```python
from build123d import *

# Parameters (mm, degrees)
F0_W      = 2.2
F0_H      = 15
F1_DEPTH  = 1.5
F0_W_2    = 4.4
F0_H_2    = 4.6
F2_DEPTH  = 15
F3_SIZE   = 12
F5_DEPTH  = 25
F6_R      = 2.85
F7_DEPTH  = 2.2
F8_R      = 1.2
F9_R      = 7.49999
F10_R     = 3.35
F11_DEPTH = 25


# Not quite as in the source:
# - a fillet or chamfer is up to 0.001 mm smaller than in the source, because OpenCascade refuses the exact size
# - a pattern or mirror of a feature is missing from the dataset's text; its kind, count and spacing are read off the source's solid


with BuildPart() as f1:
    # F0 (on Top) → F1 (new body)
    with BuildSketch(Plane.XY):
        Polygon((8.1, 0.4), (8.1, 5), (-8.1, 5), (-8.1, 0.4), (-8.1, -5), (-8.1, -20), (8.1, -20), (8.1, -5), align=None)
        with Locations((-9.2, -12.5)):
            Rectangle(F0_W, F0_H)
        with Locations((9.2, -12.5)):
            Rectangle(F0_W, F0_H)
    extrude(amount=F1_DEPTH)

    # F0 (on Top) → F2 (join)
    with BuildSketch(Plane.XY):
        with Locations((-10.3, 12.5)):
            Rectangle(F0_W_2, F0_H)
        with Locations((10.3, 12.5)):
            Rectangle(F0_W_2, F0_H)
        with Locations((-10.3, 2.7)):
            Rectangle(F0_W_2, F0_H_2)
        with Locations((10.3, 2.7)):
            Rectangle(F0_W_2, F0_H_2)
        with Locations((-11.4, -12.5)):
            Rectangle(F0_W, F0_H)
        Polygon((-8.1, -5), (-8.1, 0.4), (-12.5, 0.4), (-12.5, -5), (-10.3, -5), align=None)
        Polygon((12.5, -5), (12.5, 0.4), (8.1, 0.4), (8.1, -5), (10.3, -5), align=None)
        with Locations((11.4, -12.5)):
            Rectangle(F0_W, F0_H)
    extrude(amount=F2_DEPTH)

    # F3
    f3_edges = [f1.edges().sort_by_distance(p)[0] for p in [
        (11.4, -20, 15),
        (-11.4, -20, 15),
    ]]
    chamfer(f3_edges, length=F3_SIZE)

    # F4 (on face) → F5 (cut)
    with BuildSketch(Plane.YZ.offset(12.5)):
        Polygon((6, 12.653529644), (5, 15), (0.3, 15), (-0.7, 12.653529644), align=None)
    extrude(amount=-F5_DEPTH, mode=Mode.SUBTRACT)

    # F6 (on face) → F7 (cut)
    with BuildSketch(Plane.YZ.offset(-8.1)):
        with BuildLine():
            Line((20, 1.3383538289), (20, 13.6716461711))
            ThreePointArc((20, 13.6716461711), (19.1242226672, 14.3975416295), (18.1593630584, 15))
            Line((18.1593630584, 15), (10.1406412151, 15))
            ThreePointArc((10.1406412151, 15), (5.6500087774, 7.4943749708), (10.1593912813, 0))
            Line((10.1593912813, 0), (18.1406129922, 0))
            ThreePointArc((18.1406129922, 0), (19.1156030804, 0.6062459626), (20, 1.3383538289))
        make_face()
        with Locations((14.1500021368, 7.505)):
            Circle(F6_R, mode=Mode.SUBTRACT)
    f7 = extrude(amount=-F7_DEPTH, mode=Mode.SUBTRACT)

    # F7_copies: F7 across plane
    add(f7.mirror(Plane(origin=(0, 0, 0), x_dir=(0, 0, 1), z_dir=(1, 0, 0))), mode=Mode.SUBTRACT)

    # F8
    f8_edges = [f1.edges().sort_by_distance(p)[0] for p in [
        (-8.1, 11.300002, 7.505),
        (8.1, 11.300002, 7.505),
    ]]
    fillet(f8_edges, radius=F8_R)

    # F9 (radius 7.5 in the source; OpenCascade refuses exactly that, so slightly less here)
    f9_edges = [f1.edges().sort_by_distance(p)[0] for p in [
        (-10.3, 20, 15),
        (-10.3, 20, 0),
        (10.3, 20, 15),
        (10.3, 20, 0),
    ]]
    fillet(f9_edges, radius=F9_R)

    # F10 (on face) → F11 (cut)
    with BuildSketch(Plane.XY.offset(1.5)):
        with Locations((0, -12)):
            Circle(F10_R)
    extrude(amount=-F11_DEPTH, mode=Mode.SUBTRACT)


solid = f1.part
```
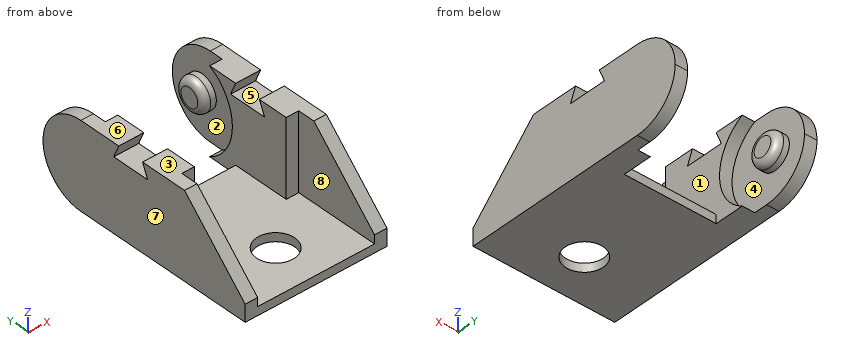
Check sheet for the modelled part. Datum: model origin and axes. Units: mm. Face numbers are marked on the shaded views. A direction names the side the tool comes from. Coordinates: 2 decimals unless noted, no trailing zeros. Loops run counter-clockwise (first coordinate to the right, second up) from the corner with the lowest first, then second, coordinate; pieces in that order, holes last.
1) Sectioned sample at B-B (y = -2.5). Record the boundary of the cut face in (x, z), and give its area (3 significant figures).
2) Sectioned sample at A-A (x = 0). Record the boundary of the cut face in (y, z).
3) Material ranges on probe 1 along X at (y, z) = (-9, 7.5); probe 2 along Y at (x, z) = (0, 1.05); probe 3 along X at (y, z) = (0.5, 6), recorded low to high.
4) Access from +Z, -Z, +X, -X, +Y, -Y to the whole of each face (thin tool, end or side, straight path). Record for the marked faces 4, 5, 6, 7 and 8.
5) Sectioned sample at D-D (y = -12). Record the boundary of the cut face in (x, z), and give its area (4 significant figures).
6) Gauge pin test, flat ends, axial feed: pin 1 (1.5 mm diameter, centred on x = 5.5, y = -0.5, fed in from +Z); pin 2 (1.3 mm diameter, centred on x = -10, y = 3, fed in from +Z); pin 3 (1.1 mm diameter, centred on x = -9.5, z = 7, fed in from -Y). Record the tip position at first contact, or that the pin passes through.
7) Release check for a two-part mould opening along Z. For the marked faces 1, 2 and 3 record: released by +Z, released by -Z, zero draft, split by the parting line, or undercut.
8) Sectioned sample at C-C (z = 2.25). Record the boundary of the cut face in (x, y), and give its area (3 significant figures).
Check sheet entries:
1. outline: (-12.5, 0) - (12.5, 0) - (12.5, 15) - (8.1, 15) - (8.1, 1.5) - (-8.1, 1.5) - (-8.1, 15) - (-12.5, 15) - close
1. area: 156 mm2
2. outline: (-20, 0) - (-15.35, 0) - (-15.35, 1.5) - (-20, 1.5) - close; (-8.65, 0) - (5, 0) - (5, 1.5) - (-8.65, 1.5) - close
3. probe 1: x = -12.5 to -10.3, 10.3 to 12.5
3. probe 2: y = -20 to -15.35, -8.65 to 5
3. probe 3: x = -12.5 to -8.1, 8.1 to 12.5
4. face 4: none
4. face 5: +X, -X
4. face 6: +Z, +X, -X, +Y, -Y
4. face 7: +Z, -Z, -X, +Y, -Y
4. face 8: +Z, -Y
5. outline: (-12.5, 0) - (-3.35, 0) - (-3.35, 1.5) - (-10.3, 1.5) - (-10.3, 11) - (-12.5, 11) - close; (3.35, 0) - (12.5, 0) - (12.5, 11) - (10.3, 11) - (10.3, 1.5) - (3.35, 1.5) - close
5. area: 69.25 mm2
6. pin 1: stops at z = 1.5
6. pin 2: stops at z = 12.65
6. pin 3: stops at y = -5
7. face 1: zero draft
7. face 2: undercut
7. face 3: released by +Z
8. outline: (-12.5, -20) - (-10.3, -20) - (-10.3, -5) - (-8.1, -5) - (-8.1, 7.47) - (-10.3, 7.47) - (-10.3, 17.86) - (-12.5, 17.86) - close; (8.1, -5) - (10.3, -5) - (10.3, -20) - (12.5, -20) - (12.5, 17.86) - (10.3, 17.86) - (10.3, 7.47) - (8.1, 7.47) - close
8. area: 221 mm2
